Can you work these out from the model? Positions are in its coordinate system, mm. Give positions to 0.01 mm unless a question says otherwise; leave off trailing zeros. Order: outer loops, then holes, each group sorted by start corner. A loop starts at its lowest first (then second) coordinate and runs counter-clockwise, first axis right, second up. Notation, with made-up numbers: M -3,45.25 L 54,45.25 A30 ccw 54,79.25 Z; hole C 30.5,-25.75 d1. An arc over 180 degrees is marked long. One line per question, with ' | ' between items. Start each with the question number.
1) I'm going to push flat-ended pins straight in: pin 1 Ø1 at (x, y) = (1.5, 23) entering from -Z; pin 2 Ø6 at (y, z) = (20.5, -9) entering from -X; pin 3 Ø1 at (x, y) = (1.5, 26.5) entering from +Z. Where does each tip first touch, or does it pass through?
2) Please list where these lines run through material, in increasing order: line 1 along Z through (x, y) = (10.25, 5); line 2 along Z through (x, y) = (5.75, 17); line 3 along X through (y, z) = (9.5, -2.75). Write a range as [from, to].
3) If we section it at B-B, the plane z = -9.75: Please give me the cut outline in (x, y), plus the area to 3 significant figures.
4) If we section it at A-A, the plane y = 29: Please give me the cut outline in (x, z), plus the area to 3 significant figures.
```python
from build123d import *

# Parameters (mm, degrees)
SKETCH1_R           = 12.7
BOSS_EXTRUDE1_DEPTH = 38.1


with BuildPart() as part:
    # Sketch1 → Boss-Extrude1 (new body)
    with BuildSketch(Plane(origin=(0, 0, 0), x_dir=(1, 0, 0), z_dir=(0, 1, 0))):
        Circle(SKETCH1_R)
    extrude(amount=BOSS_EXTRUDE1_DEPTH)

    # Sketch2 → Cut-Revolve1 (revolve, cut)
    with BuildSketch(Plane(origin=(12.7, 0, 0), x_dir=(0, 0, -1), z_dir=(1, 0, 0))):
        with BuildLine():
            Line((-12.7, 38.1), (12.7, 38.1))
            ThreePointArc((12.7, 38.1), (0, 30.707213599), (-12.7, 38.1))
        make_face()
    revolve(axis=Axis((12.7, 38.1, 12.7), (0, 0, -1)), mode=Mode.SUBTRACT)

    # Sketch3 → Cut-Revolve2 (revolve, cut)
    with BuildSketch(Plane(origin=(12.7, 0, 0), x_dir=(0, 0, -1), z_dir=(1, 0, 0))):
        with BuildLine():
            Line((-12.7, 0), (12.7, 0))
            ThreePointArc((12.7, 0), (0, 7.392786401), (-12.7, 0))
        make_face()
    revolve(axis=Axis((12.7, 0, 12.7), (0, 0, -1)), mode=Mode.SUBTRACT)

    # Sketch4 → Cut-Revolve3 (revolve, cut)
    with BuildSketch(Plane(origin=(-12.7, 0, 0), x_dir=(0, 0, -1), z_dir=(1, 0, 0))):
        with BuildLine():
            Line((-12.7, 38.1), (12.7, 38.1))
            ThreePointArc((12.7, 38.1), (0, 30.707213599), (-12.7, 38.1))
        make_face()
    revolve(axis=Axis((-12.7, 38.1, 12.7), (0, 0, -1)), mode=Mode.SUBTRACT)

    # Sketch5 → Cut-Revolve4 (revolve, cut)
    with BuildSketch(Plane(origin=(-12.7, 0, 0), x_dir=(0, 0, -1), z_dir=(1, 0, 0))):
        with BuildLine():
            Line((-12.7, 0), (12.664915911, 0))
            ThreePointArc((12.664915911, 0), (-0.017542044, 7.361983694), (-12.7, 0))
        make_face()
    revolve(axis=Axis((-12.7, 0, 0), (0, 0, 1)), mode=Mode.SUBTRACT)


solid = part.part
```
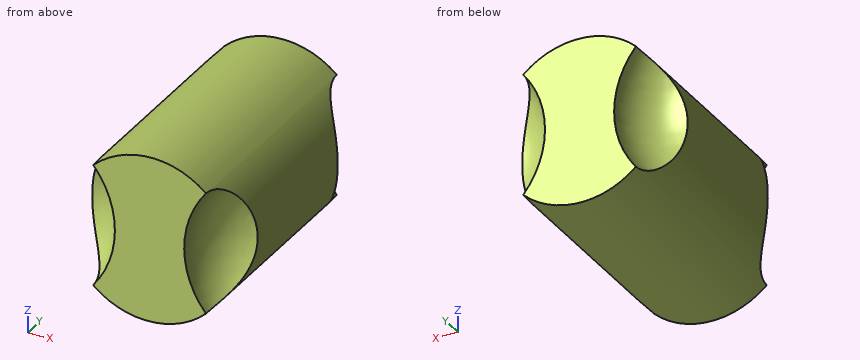
Results found:
1) pin 1: stops at z = -12.66 | pin 2: stops at x = -11.19 | pin 3: stops at z = 12.66
2) line 1: z = [-7.5, -7.07], [7.07, 7.5] | line 2: z = [-11.32, 11.32] | line 3: x = [-12.4, 12.4]
3) outline: M -8.14,0 L 8.14,0 L 8.14,38.1 L -8.14,38.1 Z | area: 620 mm²
4) outline: C 0,0 d25.4 | area: 507 mm²
